Read the model definition and answer for the solid it produces. Units are mm, in the model's axes. Round coordinates to 2 decimals unless told otherwise and drop trailing zeros. Write each loop counter-clockwise with the first axis right and the second up, starting at its lowest first coordinate (ties: lowest second). Pieces come first, ordered by that corner, then holes. Notation, with made-up numbers: (69.5, 33) -> (92.5, 33) arc R23 ccw to (92.5, 62) -> close; hole circle Ø5 at (76, 67). An arc over 180 degrees is marked (long way). Return JSON: item names as keys, results as strings. Group by question number.
(1) The mould has two halves that part along X. Classify faces 1 (the flat face through (113, 2.6, 57)), 2 (the cylindrical face through (9.333, 1.282, 141.694)), 3 (the cylindrical face through (225.59, 1.32, 2.85)), 4 (the cylindrical face through (9.333, 1.282, 12.154)): released by +X, released by -X, zero draft, split by the parting line, or undercut.
(2) A cutting plane is placed at C-C on y = 1.9. State how many separate pieces and enclosed holes the cut face has, then the cut area to 3 significant figures.
(3) A cutting plane is placed at B-B on x = 5.08. Give the vertices of the cut face in (y, z).
(4) Straight lines are drawn through the part: line 1 (X direction, y = 2.35, z = 58.5); line 2 (X direction, y = 0.8, z = 101); line 3 (Z direction, x = 144.5, y = 1.4). For each, find the intervals that lie inside material, in ascending order.
(5) Given pin 1 (0.8 mm diameter, centred on y = 1.5, z = 140.5, fed in from -X); pin 2 (2.5 mm diameter, centred on x = 218.44, z = 139.7, fed in from +Y), each flat-ended and moving along its own axis, determine where each tip first touches the part or whether it passes through.
(6) A cutting plane is placed at A-A on x = 199.5. Give the vertices of the cut face in (y, z).
```python
from build123d import *

# Parameters (mm, degrees)
SKETCH1_W           = 228.6
SKETCH1_H           = 149.86
SKETCH1_R           = 3.05
SKETCH1_R_2         = 2.159
SKETCH1_W_2         = 25.4
SKETCH1_H_2         = 3.175
BOSS_EXTRUDE1_DEPTH = 2.6
FILLET1_R           = 10
SKETCH25_W          = 104.14
SKETCH25_H          = 22.86
SKETCH25_W_2        = 3.2385
SKETCH25_H_2        = 12.7
CUT_EXTRUDE18_DEPTH = 10.16
SKETCH26_W          = 25.35893358
SKETCH26_H          = 16.469313419
CUT_EXTRUDE19_DEPTH = 7.62
SKETCH27_R          = 3
CUT_EXTRUDE20_DEPTH = 7.62


with BuildPart() as part:
    # Sketch1 → Boss-Extrude1 (new body)
    with BuildSketch(Plane(origin=(0, 0, 0), x_dir=(1, 0, 0), z_dir=(0, 1, 0))):
        with Locations((114.3, -74.93)):
            Rectangle(SKETCH1_W, SKETCH1_H)
        with Locations(Location((5.08, -58.039, 0), (0, 0, 270))):
            Circle(SKETCH1_R, mode=Mode.SUBTRACT)
        with Locations(Location((5.08, -91.821, 0), (0, 0, 270))):
            Circle(SKETCH1_R, mode=Mode.SUBTRACT)
        with Locations(Location((223.52, -91.821, 0), (0, 0, 270))):
            Circle(SKETCH1_R, mode=Mode.SUBTRACT)
        with Locations(Location((223.52, -58.039, 0), (0, 0, 270))):
            Circle(SKETCH1_R, mode=Mode.SUBTRACT)
        with Locations(Location((218.44, -10.16, 0), (0, 0, 270))):
            Circle(SKETCH1_R_2, mode=Mode.SUBTRACT)
        with Locations(Location((10.16, -10.16, 0), (0, 0, 270))):
            Circle(SKETCH1_R_2, mode=Mode.SUBTRACT)
        with Locations(Location((218.44, -139.7, 0), (0, 0, 270))):
            Circle(SKETCH1_R_2, mode=Mode.SUBTRACT)
        with Locations(Location((10.16, -139.7, 0), (0, 0, 270))):
            Circle(SKETCH1_R_2, mode=Mode.SUBTRACT)
        with Locations((35.56, -9.887961988)):
            Rectangle(SKETCH1_W_2, SKETCH1_H_2, mode=Mode.SUBTRACT)
        with Locations((193.04, -9.887961988)):
            Rectangle(SKETCH1_W_2, SKETCH1_H_2, mode=Mode.SUBTRACT)
        with Locations((193.04, -139.972038012)):
            Rectangle(SKETCH1_W_2, SKETCH1_H_2, mode=Mode.SUBTRACT)
        with Locations((35.56, -139.972038012)):
            Rectangle(SKETCH1_W_2, SKETCH1_H_2, mode=Mode.SUBTRACT)
    extrude(amount=BOSS_EXTRUDE1_DEPTH)

    # Fillet1
    fillet1_edges = [part.edges().sort_by_distance(p)[0] for p in [
        (0, 1.3, 0),
        (228.6, 1.3, 0),
        (228.6, 1.3, 149.86),
        (0, 1.3, 149.86),
    ]]
    fillet(fillet1_edges, radius=FILLET1_R)

    # Sketch25 → Cut-Extrude18 (cut)
    with BuildSketch(Plane(origin=(0, 2.6, 0), x_dir=(1, 0, 0), z_dir=(0, 1, 0))):
        with Locations((114.3, -74.93)):
            Rectangle(SKETCH25_W, SKETCH25_H)
        with Locations((10.991446919, -53.364023976)):
            Rectangle(SKETCH25_W_2, SKETCH25_H_2)
        with Locations((58.908546919, -54.507023976)):
            Rectangle(SKETCH25_W_2, SKETCH25_H_2)
        with Locations((15.741246919, -105.294323976)):
            Rectangle(SKETCH25_W_2, SKETCH25_H_2)
        with Locations((43.668546919, -105.294323976)):
            Rectangle(SKETCH25_W_2, SKETCH25_H_2)
    extrude(amount=-CUT_EXTRUDE18_DEPTH, mode=Mode.SUBTRACT)

    # Sketch26 → Cut-Extrude19 (cut)
    with BuildSketch(Plane(origin=(0, 2.6, 0), x_dir=(1, 0, 0), z_dir=(0, 1, 0))):
        with Locations((80.126817751, -46.853769114)):
            Rectangle(SKETCH26_W, SKETCH26_H)
        with Locations((80.126817751, -103.006230887)):
            Rectangle(SKETCH26_W, SKETCH26_H)
        with Locations((148.473182249, -103.006230887)):
            Rectangle(SKETCH26_W, SKETCH26_H)
        with Locations((148.473182249, -46.853769114)):
            Rectangle(SKETCH26_W, SKETCH26_H)
    extrude(amount=-CUT_EXTRUDE19_DEPTH, mode=Mode.SUBTRACT)

    # Sketch27 → Cut-Extrude20 (cut)
    with BuildSketch(Plane(origin=(0, 2.6, 0), x_dir=(1, 0, 0), z_dir=(0, 1, 0))):
        with Locations(Location((10.356901739, -26.58723359, 0), (0, 0, 270))):
            Circle(SKETCH27_R)
    extrude(amount=-CUT_EXTRUDE20_DEPTH, mode=Mode.SUBTRACT)


solid = part.part
```
Checks:
{
 "1": {"face 1": "zero draft", "face 2": "undercut", "face 3": "released by +X", "face 4": "undercut"},
 "2": {"separate pieces": "1", "enclosed holes": "22", "area": "29,400 mm^2"},
 "3": {"outline": "(0, 1.29) -> (2.6, 1.29) -> (2.6, 54.99) -> (0, 54.99) -> close; (0, 61.09) -> (2.6, 61.09) -> (2.6, 88.77) -> (0, 88.77) -> close; (0, 94.87) -> (2.6, 94.87) -> (2.6, 148.57) -> (0, 148.57) -> close"},
 "4": {"line 1": "x = 0 to 2.07, 8.09 to 9.37, 12.61 to 57.29, 60.53 to 220.51, 226.53 to 228.6", "line 2": "x = 0 to 14.12, 17.36 to 42.05, 45.29 to 67.45, 92.81 to 135.79, 161.15 to 228.6", "line 3": "z = 0 to 38.62, 55.09 to 63.5, 86.36 to 94.77, 111.24 to 149.86"},
 "5": {"pin 1": "stops at x = 0", "pin 2": "passes through"},
 "6": {"outline": "(0, 0) -> (2.6, 0) -> (2.6, 8.3) -> (0, 8.3) -> close; (0, 11.48) -> (2.6, 11.48) -> (2.6, 138.38) -> (0, 138.38) -> close; (0, 141.56) -> (2.6, 141.56) -> (2.6, 149.86) -> (0, 149.86) -> close"}
}
